from build123d import *

# Parameters (mm, degrees)
CROQUIS1_R              = 38
SALIENTE_EXTRUIR2_DEPTH = 5
CROQUIS2_R              = 10
SALIENTE_EXTRUIR3_DEPTH = 100
SALIENTE_EXTRUIR4_DEPTH = 20
CROQUIS4_R              = 10
SALIENTE_EXTRUIR5_DEPTH = 80
SALIENTE_EXTRUIR6_DEPTH = 20
CROQUIS6_R              = 10
SALIENTE_EXTRUIR7_DEPTH = 80
CROQUIS7_R              = 10
CROQUIS7_R_2            = 4
CORTAR_EXTRUIR1_DEPTH   = 18


with BuildPart() as part:
    # Croquis1 → Saliente-Extruir2 (new, symmetric)
    with BuildSketch(Plane(origin=(0, 0, 0), x_dir=(0, 0, -1), z_dir=(1, 0, 0))):
        Circle(CROQUIS1_R)
    extrude(amount=SALIENTE_EXTRUIR2_DEPTH, both=True)

    # Croquis2 → Saliente-Extruir3 (add)
    with BuildSketch(Plane(origin=(5, 0, 0), x_dir=(0, 0, -1), z_dir=(1, 0, 0))):
        Circle(CROQUIS2_R)
    saliente_extruir3 = extrude(amount=SALIENTE_EXTRUIR3_DEPTH)

    # Croquis3 → Saliente-Extruir4 (add)
    with BuildSketch(Plane(origin=(105, 0, 0), x_dir=(0, 0, -1), z_dir=(1, 0, 0))):
        with BuildLine():
            Line((-9.980675877, 0.621376727), (-14.884167289, -78.139472087))
            ThreePointArc((-14.884167289, -78.139472087), (0, -95), (14.884167289, -78.139472087))
            Line((14.884167289, -78.139472087), (9.980675877, 0.621376727))
            ThreePointArc((9.980675877, 0.621376727), (0, 10), (-9.980675877, 0.621376727))
        make_face()
    extrude(amount=SALIENTE_EXTRUIR4_DEPTH)

    # Croquis4 → Saliente-Extruir5 (add)
    with BuildSketch(Plane(origin=(125, 0, 0), x_dir=(0, 0, -1), z_dir=(1, 0, 0))):
        with Locations((0, -80)):
            Circle(CROQUIS4_R)
    extrude(amount=SALIENTE_EXTRUIR5_DEPTH)

    # Simetría1: Saliente-Extruir3 across plane
    add(saliente_extruir3.mirror(Plane(origin=(0, 0, 0), x_dir=(0, 0, 1), z_dir=(1, 0, 0))))

    # Croquis5 → Saliente-Extruir6 (add)
    with BuildSketch(Plane.ZY.offset(105)):
        with BuildLine():
            Line((-14.884167289, 78.139472087), (-9.980675877, -0.621376727))
            ThreePointArc((-9.980675877, -0.621376727), (-0.001815165, -9.999999835), (9.980449639, -0.625))
            Line((9.980449639, -0.625), (14.970674459, 79.0625))
            ThreePointArc((14.970674459, 79.0625), (-0.463536411, 94.992836089), (-14.884167289, 78.139472087))
        make_face()
    extrude(amount=SALIENTE_EXTRUIR6_DEPTH)

    # Croquis6 → Saliente-Extruir7 (add)
    with BuildSketch(Plane.ZY.offset(125)):
        with Locations((0, 80)):
            Circle(CROQUIS6_R)
    extrude(amount=SALIENTE_EXTRUIR7_DEPTH)

    # Croquis7 → Cortar-Extruir1 (cut)
    with BuildSketch(Plane(origin=(39.44, 0, 0), x_dir=(0, 0, -1), z_dir=(1, 0, 0))):
        Circle(CROQUIS7_R)
        Circle(CROQUIS7_R_2, mode=Mode.SUBTRACT)
    extrude(amount=-CORTAR_EXTRUIR1_DEPTH, mode=Mode.SUBTRACT)


solid = part.part
For this review, take the finished solid that the model builds, in its own axes (mm). A direction names the side the tool comes from. Round coordinates to 2 decimals unless told otherwise and drop trailing zeros. Write each loop counter-clockwise with the first axis right and the second up, starting at its lowest first coordinate (ties: lowest second). Pieces come first, ordered by that corner, then holes. Notation, with made-up numbers: (77, 74.5) -> (100, 74.5) arc R11 ccw to (100, 95.5) -> close; hole circle Ø10 at (46, 77). An arc over 180 degrees is marked (long way). Put each result on its own line as item: value.
Q1. To check wall thickness, follow L1, parallel to X at y = -33, z = 3; L2, parallel to X at y = 8, z = -25; L3, parallel to X at y = 18.5, z = -7.5. State the ranges of each line that lie inside material, in increasing order. Write a range as [from, to].
Determined:
L1: x = [-5, 5], [105, 125]
L2: x = [-5, 5]
L3: x = [-125, -105], [-5, 5]
Q2. The part is to be moulded in two halves that separate along X. For faces 1 (the flat face through (5, -8, -8)), 2 (the cylindrical face through (-164.44, 89.915, -1.302)), 3 (the flat face through (-205, 80, 0)), say which applies: released by +X, released by -X, zero draft, split by the parting line, or undercut.
Determined:
face 1: undercut
face 2: zero draft
face 3: released by -X
Q3. Consider section B-B on x = 10. State the section outline as (y, z) points.
Determined:
outline: circle Ø20 at (0, 0)
Q4. Machinability: for faces 4 (the flat face through (-5, -8, -8)), 5 (the flat face through (-114.86, 39.31, -12.467)), 6 (the flat face through (-114.86, 38.66, 12.44)), 7 (the flat face through (114.86, -39.31, -12.467)), which of the approach directions +Z, -Z, +X, -X, +Y, -Y give a long, thin tool a straight path to every point of the face, cutting with its end or side? Answer none if there is none.
Determined:
face 4: none
face 5: -Z, -X, -Y
face 6: +Z, -X, -Y
face 7: -Z, +X, +Y
Q5. Clearance check with flat-ended pins moving along their axes: pin 1 Ø5 at (x, z) = (-48.5, -8.5) entering from -Y; pin 2 Ø1 at (x, z) = (-82.5, 9.5) entering from -Y; pin 3 Ø1 at (x, z) = (-41, -3) entering from -Y. State where each tip first meets the part, or that it passes through.
Determined:
pin 1: stops at y = -8
pin 2: stops at y = -4.36
pin 3: stops at y = -9.68
